Work out the finished part from the listing and answer in its coordinate system (mm). A direction names the side the tool comes from. Round coordinates to 2 decimals unless told otherwise and drop trailing zeros. Write each loop counter-clockwise with the first axis right and the second up, starting at its lowest first coordinate (ties: lowest second). Pieces come first, ordered by that corner, then holes. Notation, with made-up numbers: (68, 58.5) -> (126, 58.5) arc R7 cw to (126, 70.5) -> close; hole circle Ø8 at (-24, 56). An arc over 180 degrees is marked (long way). One line per item, written item: value.
```python
from build123d import *

# Parameters (mm, degrees)
F1_DEPTH       = 9.525
F3_D           = 3.81
F3_CSINK_D     = 6.35
F3_CSINK_ANGLE = 60
F5_DEPTH       = 9.525
F5_DEPTH_BACK  = 1.5875
F7_DEPTH       = 25.4


with BuildPart() as f1:
    # F0 (on Front) → F1 (new body)
    with BuildSketch(Plane.XZ):
        with BuildLine():
            ThreePointArc((0, 19.05), (-4.259709, 20.055581), (-7.62, 22.86))
            ThreePointArc((-7.62, 22.86), (-18.379613, 21.889806), (-12.7, 12.7))
            Line((-12.7, 12.7), (12.7, 12.7))
            Line((12.7, 12.7), (12.7, -12.7))
            ThreePointArc((12.7, -12.7), (21.889806, -18.379613), (22.86, -7.62))
            ThreePointArc((22.86, -7.62), (20.055581, -4.259709), (19.05, 0))
            Line((19.05, 0), (19.05, 6.35))
            ThreePointArc((19.05, 6.35), (20.055581, 10.609709), (22.86, 13.97))
            ThreePointArc((22.86, 13.97), (23.540128, 23.540128), (13.97, 22.86))
            ThreePointArc((13.97, 22.86), (10.609709, 20.055581), (6.35, 19.05))
            Line((6.35, 19.05), (0, 19.05))
        make_face()
    extrude(amount=F1_DEPTH)

    # F3 (through all)
    with Locations(Plane.XZ.offset(9.525)):
        with Locations((-12.7, 19.05), (19.05, 19.05), (19.05, -12.7)):
            CounterSinkHole(F3_D / 2, F3_CSINK_D / 2, counter_sink_angle=F3_CSINK_ANGLE)

    # F4 (on Front) → F5 (join, two sides)
    with BuildSketch(Plane.XZ) as f5_sk:
        with BuildLine():
            Line((12.7, -12.7), (12.7, 12.7))
            Line((12.7, 12.7), (-12.7, 12.7))
            ThreePointArc((-12.7, 12.7), (-15.13004, 13.183365), (-17.190128, 14.559872))
            Line((-17.190128, 14.559872), (14.559872, -17.190128))
            ThreePointArc((14.559872, -17.190128), (13.183365, -15.13004), (12.7, -12.7))
        make_face()
    extrude(amount=F5_DEPTH)
    extrude(f5_sk.sketch, amount=-F5_DEPTH_BACK)

    # F6 (on face) → F7 (cut)
    with BuildSketch(Plane(origin=(0, 0, 0), x_dir=(-1, 0, 0), z_dir=(0, 1, 0))):
        Polygon((-12.7, -24.797732), (-12.7, -12.7), (-12.7, 12.7), (12.7, 12.7), (24.978289, 12.7), (24.821575, 21.179355), (-31.780545, 20.13324), (-31.780545, -24.797732), align=None)
    extrude(amount=F7_DEPTH, mode=Mode.SUBTRACT)


solid = f1.part
```
(1) A tool of negligible diameter and unlimited length cuts with its end or side. For faces 1 (the face through (20.028, -4.696, 10.554)), 2 (the face through (-16.75, -4.7, 23.94)), 3 (the face through (3, -5, 19.05)), 4 (the face through (-1, 1, 12.7)), from which of +Z, -Z, +X, -X, +Y, -Y can it reach the whole face along a straight path? Write none if from no direction.
Reported:
face 1: +X, +Y, -Y
face 2: +Y, -Y
face 3: +Z, +Y, -Y
face 4: +Z, +X, -X, +Y
(2) Find section A-A on y = -0.75. Give the vertices of the cut face in (x, z) (3 decimals).
Reported:
outline: (-17.19, 14.56) -> (14.56, -17.19) arc R6.35 ccw (long way) to (22.86, -7.62) arc R9.525 cw to (19.05, 0) -> (19.05, 6.35) arc R9.525 cw to (22.86, 13.97) arc R6.35 ccw (long way) to (13.97, 22.86) arc R9.525 cw to (6.35, 19.05) -> (0, 19.05) arc R9.525 cw to (-7.62, 22.86) arc R6.35 ccw (long way) to start; hole circle Ø3.81 at (-12.7, 19.05); hole circle Ø3.81 at (19.05, -12.7); hole circle Ø3.81 at (19.05, 19.05)
(3) For a pull along X with two mould halves and no side action, classify faces 5 (the face through (23.75, -4.7, -16.97)), 6 (the face through (-4.204, -4.696, 20.028)), 7 (the face through (12.7, 1, -2)), 8 (the face through (-1.54, -4.05, -1.09)) as pulls with the +X half, pulls with the -X half, needs draft (parallel to the pull), parting line crosses it, or undercut.
Reported:
face 5: parting line crosses it
face 6: undercut
face 7: pulls with the +X half
face 8: pulls with the -X half
(4) Flat-ended cylindrical pins translate along their axes: pin 1 Ø5 at (x, z) = (-12.7, 19.05) entering from -Y; pin 2 Ø1.3 at (y, z) = (0.5, 5) entering from +X; pin 3 Ø6 at (y, z) = (-2.5, -8) entering from -X; pin 4 Ø3 at (x, z) = (19.05, 19.05) entering from +Y. Find the tip coordinate at first contact, or state that the pin passes through.
Reported:
pin 1: stops at y = -8.36
pin 2: stops at x = 19.05
pin 3: stops at x = 2.37
pin 4: passes through
(5) Consider probe 1 along X at (y, z) = (-2, 18.5); probe 2 along Z at (x, y) = (-12.7, -5) (3 decimals); probe 3 along X at (y, z) = (-8.75, -13.5). Determine where each line is inside the solid, lowest interval first.
Reported:
probe 1: x = -19.03 to -14.52, -10.88 to 17.23, 20.87 to 25.38
probe 2: z = 10.07 to 17.145, 20.955 to 25.4
probe 3: x = 10.87 to 16.44, 21.66 to 25.35
(6) Find section B-B on z = -12.7. Give the vertices of the cut face in (x, y) (1 decimal).
Reported:
outline: (10.1, -9.5) -> (15.9, -9.5) -> (17.1, -7.3) -> (17.1, 0) -> (12.7, 0) -> (12.7, 1.6) -> (10.1, 1.6) -> close; (21, -7.3) -> (22.2, -9.5) -> (25.4, -9.5) -> (25.4, 0) -> (21, 0) -> close
(7) Find section C-C on x = -12.7. Give the vertices of the cut face in (y, z) (1 decimal), plus the area to 3 significant figures.
Reported:
outline: (-9.5, 10.1) -> (1.6, 10.1) -> (1.6, 12.7) -> (0, 12.7) -> (0, 17.1) -> (-7.3, 17.1) -> (-9.5, 15.9) -> close; (-9.5, 22.2) -> (-7.3, 21) -> (0, 21) -> (0, 25.4) -> (-9.5, 25.4) -> close
area: 111 mm2
